```python
from build123d import *

# Parameters (mm, degrees)
SKETCH002_R                = 11.5
SKETCH002_R_2              = 10.5
EXTRUDE005_DEPTH           = 1
EXTRUDE004_DEPTH           = 3
EXTRUDE004_PLACEMENT_ANGLE = 90
EXTRUDE002_DEPTH           = 3
EXTRUDE002_PLACEMENT_ANGLE = 90
EXTRUDE001_DEPTH           = 3
EXTRUDE003_DEPTH           = 3
EXTRUDE003_PLACEMENT_ANGLE = 180
SKETCH_R                   = 11.5
SKETCH_R_2                 = 1
SKETCH_R_3                 = 3
EXTRUDE_DEPTH              = 3
FILLET_R                   = 1.49
CHAMFER_SIZE               = 0.5
CHAMFER001_SIZE            = 0.5


with BuildPart() as extrude005:
    # Sketch002 (on Face4 of Cut) → Extrude005 (new body)
    with BuildSketch(Plane.XY.offset(3)):
        Circle(SKETCH002_R)
        Circle(SKETCH002_R_2, mode=Mode.SUBTRACT)
    extrude(amount=-EXTRUDE005_DEPTH)


with BuildPart() as extrude004:
    # Sketch001 (on Face7 of Extrude) → Extrude004 (new body)
    with BuildSketch(Plane(origin=(0, 0, 0), x_dir=(1, 0, 0), z_dir=(0, 0, -1))):
        Polygon((-11.970047, 4.898979), (-4.242641, 2.828427), (-2.828427, 4.242641), (-4.898979, 11.970047), align=None)
    extrude(amount=-EXTRUDE004_DEPTH)


with BuildPart() as extrude004_1:
    # Extrude004 placement: moved
    add(extrude004.part.rotate(Axis((0, 0, 0), (0, 0, -1)), EXTRUDE004_PLACEMENT_ANGLE))


with BuildPart() as extrude002:
    # Sketch001 (on Face7 of Extrude) → Extrude002 (new body)
    with BuildSketch(Plane(origin=(0, 0, 0), x_dir=(1, 0, 0), z_dir=(0, 0, -1))):
        Polygon((-11.970047, 4.898979), (-4.242641, 2.828427), (-2.828427, 4.242641), (-4.898979, 11.970047), align=None)
    extrude(amount=-EXTRUDE002_DEPTH)


with BuildPart() as extrude002_1:
    # Extrude002 placement: moved
    add(extrude002.part.rotate(Axis((0, 0, 0), (0, 0, 1)), EXTRUDE002_PLACEMENT_ANGLE))


with BuildPart() as extrude001:
    # Sketch001 (on Face7 of Extrude) → Extrude001 (new body)
    with BuildSketch(Plane(origin=(0, 0, 0), x_dir=(1, 0, 0), z_dir=(0, 0, -1))):
        Polygon((-11.970047, 4.898979), (-4.242641, 2.828427), (-2.828427, 4.242641), (-4.898979, 11.970047), align=None)
    extrude(amount=-EXTRUDE001_DEPTH)


with BuildPart() as fusion:
    # Sketch001 (on Face7 of Extrude) → Extrude003 (new body)
    with BuildSketch(Plane(origin=(0, 0, 0), x_dir=(1, 0, 0), z_dir=(0, 0, -1))):
        Polygon((-11.970047, 4.898979), (-4.242641, 2.828427), (-2.828427, 4.242641), (-4.898979, 11.970047), align=None)
    extrude(amount=-EXTRUDE003_DEPTH)


with BuildPart() as fusion_1:
    # Extrude003 placement: moved
    add(fusion.part.rotate(Axis((0, 0, 0), (0, 0, 1)), EXTRUDE003_PLACEMENT_ANGLE))

    # Fusion: union Extrude004, Extrude002, Extrude001
    add(extrude004_1.part)
    add(extrude002_1.part)
    add(extrude001.part)


with BuildPart() as fusion002:
    # Sketch → Extrude (new body)
    with BuildSketch(Plane.XY):
        Circle(SKETCH_R)
        with Locations((0, 6)):
            Circle(SKETCH_R_2, mode=Mode.SUBTRACT)
        with Locations((-8, 0)):
            Circle(SKETCH_R_2, mode=Mode.SUBTRACT)
        with Locations((0, -6)):
            Circle(SKETCH_R_2, mode=Mode.SUBTRACT)
        with Locations((8, 0)):
            Circle(SKETCH_R_2, mode=Mode.SUBTRACT)
        Circle(SKETCH_R_3, mode=Mode.SUBTRACT)
    extrude(amount=EXTRUDE_DEPTH)

    # Cut: cut Fusion
    add(fusion_1.part, mode=Mode.SUBTRACT)

    # Fillet
    fillet_edges = [fusion002.edges().sort_by_distance(p)[0] for p in [
        (4.242641, 2.828427, 1.5),
        (4.242641, -2.828427, 1.5),
        (2.828427, -4.242641, 1.5),
        (-2.828427, -4.242641, 1.5),
        (-4.242641, -2.828427, 1.5),
        (-4.242641, 2.828427, 1.5),
        (-2.828427, 4.242641, 1.5),
        (2.828427, 4.242641, 1.5),
    ]]
    fillet(fillet_edges, radius=FILLET_R)

    # Chamfer
    chamfer_edges = [fusion002.edges().sort_by_distance(p)[0] for p in [
        (7.823063, -3.787798, 0),
        (4.302299, -3.051077, 0),
        (3.535534, -3.535534, 0),
        (3.051077, -4.302299, 0),
        (7.823063, 3.787798, 0),
        (3.787798, -7.823063, 0),
        (4.302299, 3.051077, 0),
        (3.535534, 3.535534, 0),
        (-3.787798, -7.823063, 0),
        (3.051077, 4.302299, 0),
        (-3.051077, -4.302299, 0),
        (3.787798, 7.823063, 0),
        (-3.535534, -3.535534, 0),
        (-4.302299, -3.051077, 0),
        (-3.787798, 7.823063, 0),
        (-7.823063, -3.787798, 0),
        (-3.051077, 4.302299, 0),
        (-3.535534, 3.535534, 0),
        (-7.823063, 3.787798, 0),
        (-4.302299, 3.051077, 0),
    ]]
    chamfer(chamfer_edges, length=CHAMFER_SIZE)

    # Chamfer001
    chamfer001_edges = [fusion002.edges().sort_by_distance(p)[0] for p in [
        (11.313619, -2.062044, 0),
        (11.313619, 2.062044, 0),
        (0, -11.5, 0),
        (0, 11.5, 0),
        (-11.5, 0, 0),
    ]]
    chamfer(chamfer001_edges, length=CHAMFER001_SIZE)

    # Fusion002: union Extrude005
    add(extrude005.part)


solid = fusion002.part
```
Source: CAD feature listing. Evaluate the final solid. Frame: model axes, mm. A direction names the side the tool comes from. Give positions to 0.01 mm unless a question says otherwise; leave off trailing zeros. Loops run counter-clockwise (first coordinate to the right, second up) from the corner with the lowest first, then second, coordinate; pieces in that order, holes last. Notation, with made-up numbers: (47, -10.75) -> (60, -10.75) arc R32 ccw to (60, 24.25) -> close; hole circle Ø5 at (68, 24). An arc over 180 degrees is marked (long way). Put each result on its own line as item: value. Start each with the question number.
1) Cut plane A-A (z = 2.45). State how many separate pieces and enclosed holes the cut face has, then the cut area to 3 significant figures.
2) Cut plane D-D (y = 6). Return loops of the section in (x, z).
3) Material intervals for probe 1 along Y at (x, z) = (0, 2.3); probe 2 along Y at (x, z) = (4.75, 2.4); probe 3 along X at (y, z) = (-0.5, 2.65), sorted ascending.
4) Contact query for flat-ended pins moving along their axis: P1, Ø1.5, axis at x = -8.5, z = 0.5, coming from the -Y side; P2, Ø1.9, axis at x = 7.5, y = 7.5, coming from the -Z side; P3, Ø7, axis at x = -7, y = -7, coming from the -Z side. Output: stop coordinate, or through.
5) Draft query along X for faces 5 (the face through (-3.6, 7.9, 0.3)), 6 (the face through (7.46, 7.39, 2.51)), 7 (the face through (3.5, 7.9, 0.2)). Return one class per face: released by +X, released by -X, zero draft, split by the parting line, or undercut.
6) Reachability of faces 1 (the face through (-7.862, -3.798, 1.732)), 2 (the face through (-7.9, -3.6, 0.3)), 3 (the face through (-3.539, -7.848, 0.253)), 4 (the face through (-4.292, 3.054, 1.768)) from +Z, -Z, +X, -X, +Y, -Y: full face, straight path, thin tool, end or side. Return the list, or none.
7) Cut plane B-B (x = 0). Return loops of the section in (y, z).
Results are:
1. separate pieces: 1
1. enclosed holes: 9
1. area: 270 mm2
2. outline: (-9.81, 2) -> (-8.62, 2) -> (-8.62, 3) -> (-9.81, 3) -> close; (-3.3, 0.5) -> (-2.78, 0) -> (-1, 0) -> (-1, 3) -> (-3.3, 3) -> close; (1, 0) -> (2.78, 0) -> (3.3, 0.5) -> (3.3, 3) -> (1, 3) -> close; (8.62, 2) -> (9.81, 2) -> (9.81, 3) -> (8.62, 3) -> close
3. probe 1: y = -11.5 to -7, -5 to -3, 3 to 5, 7 to 11.5
3. probe 2: y = -10.47 to -9.36, -3 to 3, 9.36 to 10.47
3. probe 3: x = -11.49 to -8.87, -7.13 to -2.96, 2.96 to 7.13, 8.87 to 11.49
4. P1: stops at y = -4.17
4. P2: stops at z = 2
4. P3: stops at z = 0.32
5. face 5: released by -X
5. face 6: undercut
5. face 7: released by +X
6. face 1: -Z
6. face 2: -Z, -Y
6. face 3: -Z, -X
6. face 4: +Z, -Z
7. outline: (-11.5, 0.5) -> (-11, 0) -> (-7, 0) -> (-7, 3) -> (-11.5, 3) -> close; (-5, 0) -> (-3, 0) -> (-3, 3) -> (-5, 3) -> close; (3, 0) -> (5, 0) -> (5, 3) -> (3, 3) -> close; (7, 0) -> (11, 0) -> (11.5, 0.5) -> (11.5, 3) -> (7, 3) -> close
